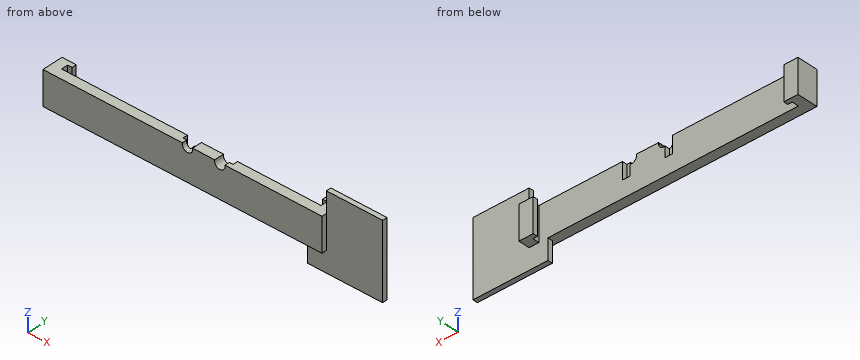
from build123d import *

# Parameters (mm, degrees)
BOSS_EXTRUDE1_DEPTH = 3.302
SKETCH2_W           = 11.43
SKETCH2_H           = 7.112
BOSS_EXTRUDE2_DEPTH = 3.302
SKETCH3_W           = 11.43
SKETCH3_H           = 7.112
BOSS_EXTRUDE3_DEPTH = 3.302
SKETCH4_W           = 1.524
SKETCH4_H           = 11.43
BOSS_EXTRUDE4_DEPTH = 1.524
SKETCH5_W           = 1.524
SKETCH5_H           = 11.43
BOSS_EXTRUDE5_DEPTH = 1.524
SKETCH7_W           = 2.54
SKETCH7_H           = 5.715
CUT_EXTRUDE1_DEPTH  = 1.651
BOSS_EXTRUDE8_START = -3.302
BOSS_EXTRUDE8_DEPTH = 1.651


with BuildPart() as part:
    # Sketch1 → Boss-Extrude1 (new body)
    with BuildSketch(Plane(origin=(0, 0, 0), x_dir=(1, 0, 0), z_dir=(0, 1, 0))):
        with BuildLine():
            Line((-29.60690112, 0), (0, 0))
            Line((0, 0), (0, 11.43))
            Line((0, 11.43), (-88.011, 11.43))
            Line((-88.011, 11.43), (-88.011, 0))
            Line((-88.011, 0), (-44.05309888, 0))
            ThreePointArc((-44.05309888, 0), (-42.508016011, 2.148644564), (-40.5384, 0.381))
            ThreePointArc((-40.5384, 0.381), (-40.548755436, 0.189383989), (-40.57970112, 0))
            Line((-40.57970112, 0), (-33.08029888, 0))
            ThreePointArc((-33.08029888, 0), (-31.535216011, 2.148644564), (-29.5656, 0.381))
            ThreePointArc((-29.5656, 0.381), (-29.575955436, 0.189383989), (-29.60690112, 0))
        make_face()
    extrude(amount=BOSS_EXTRUDE1_DEPTH)

    # Sketch2 → Boss-Extrude2 (add)
    with BuildSketch(Plane(origin=(0, 0, 0), x_dir=(0, 0, -1), z_dir=(1, 0, 0))):
        with Locations((5.715, 3.556)):
            Rectangle(SKETCH2_W, SKETCH2_H)
    extrude(amount=BOSS_EXTRUDE2_DEPTH)

    # Sketch3 → Boss-Extrude3 (add)
    with BuildSketch(Plane.ZY.offset(88.011)):
        with Locations((-5.715, 3.556)):
            Rectangle(SKETCH3_W, SKETCH3_H)
    extrude(amount=BOSS_EXTRUDE3_DEPTH)

    # Sketch4 → Boss-Extrude4 (add)
    with BuildSketch(Plane(origin=(0, 7.112, 0), x_dir=(1, 0, 0), z_dir=(0, 1, 0))):
        with Locations((-87.249, 5.715)):
            Rectangle(SKETCH4_W, SKETCH4_H)
    extrude(amount=-BOSS_EXTRUDE4_DEPTH)

    # Sketch5 → Boss-Extrude5 (add)
    with BuildSketch(Plane(origin=(0, 7.112, 0), x_dir=(1, 0, 0), z_dir=(0, 1, 0))):
        with Locations((-0.762, 5.715)):
            Rectangle(SKETCH5_W, SKETCH5_H)
    extrude(amount=-BOSS_EXTRUDE5_DEPTH)

    # Sketch7 → Cut-Extrude1 (cut)
    with BuildSketch(Plane(origin=(0, 3.302, 0), x_dir=(1, 0, 0), z_dir=(0, 1, 0))):
        with Locations((-44.05309888, 2.8575)):
            Rectangle(SKETCH7_W, SKETCH7_H)
        with Locations((-29.60690112, 2.8575)):
            Rectangle(SKETCH7_W, SKETCH7_H)
    extrude(amount=-CUT_EXTRUDE1_DEPTH, mode=Mode.SUBTRACT)

    # Sketch9 → Boss-Extrude8 (add)
    with BuildSketch(Plane.XZ.offset(BOSS_EXTRUDE8_START)):
        Polygon((-3.048, -11.43), (-3.048, -18.415), (22.352, -18.415), (22.352, 6.985), (3.302, 6.985), (3.302, 0), (3.302, -11.43), align=None)
    extrude(amount=BOSS_EXTRUDE8_DEPTH)


solid = part.part
Input: part model. Units: mm. Frame: model coordinates. Round coordinates to 2 decimals unless told otherwise and drop trailing zeros. Order: outer loops, then holes, each group sorted by start corner. A loop starts at its lowest first (then second) coordinate and runs counter-clockwise, first axis right, second up. Notation, with made-up numbers: (23.5, -32.5) - (67.5, -32.5) arc R5 ccw to (67.5, -26.5) - close; hole circle Ø4 at (73.5, -17.5). An arc over 180 degrees is marked (long way). Answer as a JSON object with one key per item and string values. Group by question number.
(1) Material intervals for probe 1 along X at (y, z) = (6.25, -1.75); probe 2 along X at (y, z) = (2.5, -3.5); probe 3 along X at (y, z) = (5, -6), sorted ascending. Write a range as from..to.
(2) Cut plane A-A (y = 4.25). Return loops of the section in (x, z).
(3) Cut plane C-C (x = -77). Return loops of the section in (y, z), then the cut area to 3 significant figures.
(4) Pin query (flat end, axial travel): P1, Ø1, axis at x = -38, z = -4.5, coming from the +Y side; P2, Ø1.3, axis at x = -44.5, y = 2.5, coming from the +Z side (3 decimals); P3, Ø0.8, axis at y = 2.5, z = -14.5, coming from the -X side; P4, Ø3, axis at x = -31.34, z = -0.38, coming from the -Y side. Return the tip coordinate at first contact, or that it passes through.
(5) Cut plane B-B (z = -9.25). Return loops of the section in (x, y), then the cut area to 3 significant figures.
Here are the results:
{
 "1": {"probe 1": "x = -91.31..-86.49, -1.52..3.3", "probe 2": "x = -91.31..-45.32, -42.78..-30.88, -28.34..22.35", "probe 3": "x = -91.31..-88.01, 0..3.3"},
 "2": {"outline": "(-91.31, -11.43) - (-88.01, -11.43) - (-88.01, 0) - (-91.31, 0) - close; (0, -11.43) - (3.3, -11.43) - (3.3, 0) - (0, 0) - close"},
 "3": {"outline": "(0, -11.43) - (3.3, -11.43) - (3.3, 0) - (0, 0) - close", "area": "37.7 mm^2"},
 "4": {"P1": "stops at y = 3.3", "P2": "stops at z = -5.715", "P3": "stops at x = -3.05", "P4": "passes through"},
 "5": {"outline": "(-91.31, 0) - (3.3, 0) - (3.3, 1.65) - (22.35, 1.65) - (22.35, 3.3) - (3.3, 3.3) - (3.3, 7.11) - (-1.52, 7.11) - (-1.52, 5.59) - (0, 5.59) - (0, 3.3) - (-88.01, 3.3) - (-88.01, 5.59) - (-86.49, 5.59) - (-86.49, 7.11) - (-91.31, 7.11) - close", "area": "374 mm^2"}
}
